```python
from build123d import *

# Parameters (mm, degrees)
ESQUISSE1_W                     = 50
ESQUISSE1_H                     = 50
BOSS_EXTRU_1_DEPTH              = 30
ESQUISSE2_W                     = 84
ESQUISSE2_H                     = 84
ENL_V_MAT_EXTRU_1_DEPTH         = 77.811457479
DIAM_TRE_DU_PER_AGE_12_0_12_1_D = 12
DIAM_TRE_DU_PER_AGE_9_0_9_2_D   = 9
CHANFREIN1_SIZE                 = 0.5
CONG_1_R                        = 3
CONG_2_R                        = 4.00000002


with BuildPart() as part:
    # Esquisse1 → Boss.-Extru.1 (new body)
    with BuildSketch(Plane.XY.offset(20.5)):
        with Locations((25, 25)):
            Rectangle(ESQUISSE1_W, ESQUISSE1_H)
    extrude(amount=-BOSS_EXTRU_1_DEPTH)

    # Esquisse2 → Enlèv. mat.-Extru.1 (cut, through all)
    with BuildSketch(Plane(origin=(0, 0, -9.5), x_dir=(-1, 0, 0), z_dir=(0, 0, -1))):
        with Locations((-48, 48)):
            Rectangle(ESQUISSE2_W, ESQUISSE2_H)
    extrude(amount=-ENL_V_MAT_EXTRU_1_DEPTH, mode=Mode.SUBTRACT)

    # Diamètre du perçage Ø12.0 (12)1 (through all)
    with Locations(Plane(origin=(0, 6, 0), x_dir=(1, 0, 0), z_dir=(0, 1, 0))):
        with Locations((30, -5.5)):
            Hole(DIAM_TRE_DU_PER_AGE_12_0_12_1_D / 2)

    # Diamètre du perçage Ø9.0 (9)2 (through all)
    with Locations(Plane(origin=(6, 0, 0), x_dir=(0, 0, -1), z_dir=(1, 0, 0))):
        with Locations((-5.5, 30)):
            Hole(DIAM_TRE_DU_PER_AGE_9_0_9_2_D / 2)

    # Chanfrein1
    chanfrein1_edges = [part.edges().sort_by_distance(p)[0] for p in [
        (36, 6, 5.5),
        (36, 0, 5.5),
        (6, 30, 1),
        (0, 30, 1),
    ]]
    chamfer(chanfrein1_edges, length=CHANFREIN1_SIZE)

    # Congé1
    cong_1_edges = [part.edges().sort_by_distance(p)[0] for p in [
        (6, 6, 5.5),
    ]]
    fillet(cong_1_edges, radius=CONG_1_R)

    # Congé2
    cong_2_edges = [part.edges().sort_by_distance(p)[0] for p in [
        (50, 6, 5.5),
        (6, 50, 5.5),
    ]]
    fillet(cong_2_edges, radius=CONG_2_R)


solid = part.part
```
Verification items for the finished model (mm, model axes). A direction names the side the tool comes from. Coordinates: 2 decimals unless noted, no trailing zeros. Loops run counter-clockwise (first coordinate to the right, second up) from the corner with the lowest first, then second, coordinate; pieces in that order, holes last. Notation, with made-up numbers: (63.25, 68) - (115.25, 68) arc R19 ccw to (115.25, 104) - close; hole circle Ø7 at (40.5, 87). An arc over 180 degrees is marked (long way). Return JSON: item names as keys, results as strings.
1. Thickness scan on L1, parallel to Y at x = 2, z = 5.5; L2, parallel to X at y = 1.5, z = 5.5; L3, parallel to Y at x = 42.5, z = 12.75. Record the ranges inside material, lowest first.
Established:
{"L1": "y = 0 to 25.5, 34.5 to 50", "L2": "x = 0 to 24, 36 to 50", "L3": "y = 0 to 6"}
2. Tool access check on faces 1 (the flat face through (6, 23, 5)), 2 (the flat face through (14, 5, 20.5)). Record the directions out of +Z, -Z, +X, -X, +Y, -Y that give a thin tool (end or side, any length) a straight path to the whole face; none if there is none.
Established:
{"face 1": "+Z, -Z, +X, +Y", "face 2": "+Z, +X, -X, +Y, -Y"}
3. Go/stop test with flat-tipped pins: pin 1 (2 mm diameter, centred on y = 13, z = 11.5, fed in from +X); pin 2 (9 mm diameter, centred on x = 27, z = 9, fed in from +Y). Record where each tip stops, or that it passes through.
Established:
{"pin 1": "stops at x = 6", "pin 2": "stops at y = 6"}
4. Section check C-C, the plane z = -7.25. Record the boundary of the cut face in (x, y).
Established:
{"outline": "(0, 0) - (50, 0) - (50, 2) arc R4 ccw to (46, 6) - (9, 6) arc R3 cw to (6, 9) - (6, 46) arc R4 ccw to (2, 50) - (0, 50) - close"}
5. Section check A-A, the plane y = 30. Record the boundary of the cut face in (x, z).
Established:
{"outline": "(0, -9.5) - (6, -9.5) - (6, 0.5) - (5.5, 1) - (0.5, 1) - (0, 0.5) - close; (0, 10.5) - (0.5, 10) - (5.5, 10) - (6, 10.5) - (6, 20.5) - (0, 20.5) - close"}
6. Section check D-D, the plane x = 21. Record the boundary of the cut face in (y, z), then the cut area to 3 significant figures.
Established:
{"outline": "(0, -9.5) - (6, -9.5) - (6, 20.5) - (0, 20.5) - close", "area": "180 mm2"}
7. Mould release check, pull along Z, two halves, no side actions. Record for faces 3 (the cylindrical face through (2.97, 25.61, 4.52)), 4 (the flat face through (14, 5, -9.5)), 5 (the cylindrical face through (6.86, 6.9, 5.71)): +Z half, -Z half, draft (parallel to the pull), parting line (faces both ways), or undercut.
Established:
{"face 3": "undercut", "face 4": "-Z half", "face 5": "draft"}
8. Section check B-B, the plane x = 30. Record the boundary of the cut face in (y, z).
Established:
{"outline": "(0, -9.5) - (6, -9.5) - (6, -1) - (5.5, -0.5) - (0.5, -0.5) - (0, -1) - close; (0, 12) - (0.5, 11.5) - (5.5, 11.5) - (6, 12) - (6, 20.5) - (0, 20.5) - close"}
